Design review of the part built by this model. Coordinates are the model's own, in mm. A direction names the side the tool comes from. Round coordinates to 2 decimals unless told otherwise and drop trailing zeros. Loops run counter-clockwise (first coordinate to the right, second up) from the corner with the lowest first, then second, coordinate; pieces in that order, holes last. Notation, with made-up numbers: (-3, 21) -> (16, 21) arc R20 ccw to (16, 52) -> close; hole circle Ø4 at (-17.75, -30). An arc over 180 degrees is marked (long way). Answer as CSV lines item,"result". Start each with the question number.
(1) Draft analysis for pull direction X (two halves, no side actions). For faces 5 (the face through (-37.82, 50.91, -0.44)), 6 (the face through (-83.683, 80.085, 1.014)), 7 (the face through (-135.546, 50, -1)), state which applies: +X half, -X half, draft (parallel to the pull), parting line (faces both ways), or undercut.
(2) Take a section at A-A, the plane x = -70. Write out the cut boundary in (y, z).
(3) Take a section at B-B, the plane z = 0.95. State how many separate pieces and enclosed holes the cut face has, and give its area (3 significant figures).
(4) Take a section at C-C, the plane x = -91.5. Write out the cut boundary in (y, z), and give its area (3 significant figures).
(5) Take a section at D-D, the plane y = 74.5. Write out the cut boundary in (x, z).
(6) To check wall thickness, follow line 1 (X direction, y = 63.5, z = -1.85); line 2 (X direction, y = 53.5, z = 1.3); line 3 (X direction, y = 65, z = 0.1). State the ranges of each line that lie inside material, in increasing order. Write a range as from..to.
(7) For P1, Ø1, axis at y = 63.5, z = -2.5, coming from the +X side; P2, Ø5.5, axis at x = -103.53, y = 78.4, coming from the +Z side; P3, Ø1, axis at x = -108.5, z = 1.5, coming from the -Y side; P4, Ø1.5, axis at x = -127.5, z = -0.5, coming from the +Y side, all flat-tipped, find the tip position at first contact; note any pin that passes through.
(8) Machinability: for faces 1 (the face through (-92, 51, 0)), 2 (the face through (-117.68, 67, -1)), 3 (the face through (-84, 76, 0)), 4 (the face through (-83.486, 51, 1)), which of the approach directions +Z, -Z, +X, -X, +Y, -Y give a long, thin tool a straight path to every point of the face, cutting with its end or side? Answer none if there is none.
from build123d import *

# Parameters (mm, degrees)
ESQUISSE1_R             = 1.7
BOSS_EXTRU_1_DEPTH      = 3
ESQUISSE2_R             = 5.2
BOSS_EXTRU_2_DEPTH      = 3
BOSS_EXTRU_2_DEPTH_BACK = 3
ESQUISSE5_W             = 129.390100882
ESQUISSE5_H             = 120.053414285
ENL_V_MAT_EXTRU_2_DEPTH = 1
ESQUISSE6_R             = 1.5
ENL_V_MAT_EXTRU_3_DEPTH = 8
ESQUISSE7_W             = 14.610679854
ESQUISSE7_H             = 62.75
ENL_V_MAT_EXTRU_4_DEPTH = 8
BOSS_EXTRU_3_DEPTH      = 7
BOSS_EXTRU_4_DEPTH      = 7
ESQUISSE11_W            = 149.051338644
ESQUISSE11_H            = 13.366564364
ENL_V_MAT_EXTRU_5_DEPTH = 80
ESQUISSE13_R            = 1.7
ENL_V_MAT_EXTRU_6_DEPTH = 15


with BuildPart() as part:
    # Esquisse1 → Boss.-Extru.1 (new body)
    with BuildSketch(Plane.XY):
        with BuildLine():
            Line((-117.680084405, 66.939310237), (-117.680084405, 59.695120061))
            ThreePointArc((-117.680084405, 59.695120061), (-116.069171702, 55.806032765), (-112.180084405, 54.195120061))
            Line((-112.180084405, 54.195120061), (-105.294175096, 54.195120061))
            ThreePointArc((-105.294175096, 54.195120061), (-101.4050878, 52.584207358), (-99.794175096, 48.695120061))
            Line((-99.794175096, 48.695120061), (-99.794175096, 35.930823665))
            ThreePointArc((-99.794175096, 35.930823665), (-101.4050878, 32.041736368), (-105.294175096, 30.430823665))
            Line((-105.294175096, 30.430823665), (-112.180084405, 30.430823665))
            ThreePointArc((-112.180084405, 30.430823665), (-116.069171702, 28.819910961), (-117.680084405, 24.930823665))
            Line((-117.680084405, 24.930823665), (-117.680084405, 23.910007682))
            ThreePointArc((-117.680084405, 23.910007682), (-116.069171702, 20.020920385), (-112.180084405, 18.410007682))
            Line((-112.180084405, 18.410007682), (-105.294175096, 18.410007682))
            ThreePointArc((-105.294175096, 18.410007682), (-101.4050878, 16.799094979), (-99.794175096, 12.910007682))
            Line((-99.794175096, 12.910007682), (-99.794175096, 1.692208933))
            ThreePointArc((-99.794175096, 1.692208933), (-101.4050878, -2.196878364), (-105.294175096, -3.807791067))
            Line((-105.294175096, -3.807791067), (-113.390601299, -3.807791067))
            ThreePointArc((-113.390601299, -3.807791067), (-117.279688595, -5.418703771), (-118.890601299, -9.307791067))
            Line((-118.890601299, -9.307791067), (-118.890601299, -18.42196685))
            ThreePointArc((-118.890601299, -18.42196685), (-117.279688595, -22.311054147), (-113.390601299, -23.92196685))
            Line((-113.390601299, -23.92196685), (-52.866544484, -23.92196685))
            ThreePointArc((-52.866544484, -23.92196685), (-48.977457187, -22.311054147), (-47.366544484, -18.42196685))
            Line((-47.366544484, -18.42196685), (-47.366544484, -9.307791067))
            ThreePointArc((-47.366544484, -9.307791067), (-48.977457187, -5.418703771), (-52.866544484, -3.807791067))
            Line((-52.866544484, -3.807791067), (-77.986378892, -3.807791067))
            ThreePointArc((-77.986378892, -3.807791067), (-81.875466189, -2.196878364), (-83.486378892, 1.692208933))
            Line((-83.486378892, 1.692208933), (-83.486378892, 12.910007682))
            ThreePointArc((-83.486378892, 12.910007682), (-81.875466189, 16.799094979), (-77.986378892, 18.410007682))
            Line((-77.986378892, 18.410007682), (-69.856378892, 18.410007682))
            ThreePointArc((-69.856378892, 18.410007682), (-65.967291596, 20.020920385), (-64.356378892, 23.910007682))
            Line((-64.356378892, 23.910007682), (-64.356378892, 24.930823665))
            ThreePointArc((-64.356378892, 24.930823665), (-65.967291596, 28.819910961), (-69.856378892, 30.430823665))
            Line((-69.856378892, 30.430823665), (-77.986378892, 30.430823665))
            ThreePointArc((-77.986378892, 30.430823665), (-81.875466189, 32.041736368), (-83.486378892, 35.930823665))
            Line((-83.486378892, 35.930823665), (-83.486378892, 55.219310237))
            ThreePointArc((-83.486378892, 55.219310237), (-81.875466189, 59.108397534), (-77.986378892, 60.719310237))
            Line((-77.986378892, 60.719310237), (-54.190366806, 60.719310237))
            ThreePointArc((-54.190366806, 60.719310237), (-50.30127951, 62.330222941), (-48.690366806, 66.219310237))
            Line((-48.690366806, 66.219310237), (-48.690366806, 67.219310237))
            Line((-48.690366806, 67.219310237), (-48.690366806, 77.901748252))
            ThreePointArc((-48.690366806, 77.901748252), (-50.30127951, 81.790835548), (-54.190366806, 83.401748252))
            Line((-54.190366806, 83.401748252), (-112.180084405, 83.401748252))
            ThreePointArc((-112.180084405, 83.401748252), (-116.069171702, 81.790835548), (-117.680084405, 77.901748252))
            Line((-117.680084405, 77.901748252), (-117.680084405, 67.219310237))
            Line((-117.680084405, 67.219310237), (-117.680084405, 66.939310237))
        make_face()
        with Locations((-59.266378892, -15.663707737)):
            Circle(ESQUISSE1_R, mode=Mode.SUBTRACT)
        with Locations((-59.266378892, 66.939310237)):
            Circle(ESQUISSE1_R, mode=Mode.SUBTRACT)
        with Locations((-91.856378892, 36.719310237)):
            Circle(ESQUISSE1_R, mode=Mode.SUBTRACT)
        with Locations((-107.466378892, -14.520689763)):
            Circle(ESQUISSE1_R, mode=Mode.SUBTRACT)
        with Locations((-107.466378892, 60.719310237)):
            Circle(ESQUISSE1_R, mode=Mode.SUBTRACT)
        with Locations((-58.306378892, 78.399310237)):
            Circle(ESQUISSE1_R, mode=Mode.SUBTRACT)
        with Locations((-108.486378892, 78.399310237)):
            Circle(ESQUISSE1_R, mode=Mode.SUBTRACT)
        with BuildLine():
            Line((-111.390601299, 21.460065469), (-70.086378892, 21.460065469))
            ThreePointArc((-70.086378892, 21.460065469), (-68.67216533, 22.045851906), (-68.086378892, 23.460065469))
            Line((-68.086378892, 23.460065469), (-68.086378892, 24.842520386))
            ThreePointArc((-68.086378892, 24.842520386), (-68.67216533, 26.256733949), (-70.086378892, 26.842520386))
            Line((-70.086378892, 26.842520386), (-111.390601299, 26.842520386))
            ThreePointArc((-111.390601299, 26.842520386), (-112.804814861, 26.256733949), (-113.390601299, 24.842520386))
            Line((-113.390601299, 24.842520386), (-113.390601299, 23.460065469))
            ThreePointArc((-113.390601299, 23.460065469), (-112.804814861, 22.045851906), (-111.390601299, 21.460065469))
        make_face(mode=Mode.SUBTRACT)
    extrude(amount=BOSS_EXTRU_1_DEPTH)

    # Esquisse2 → Boss.-Extru.2 (add, two sides)
    with BuildSketch(Plane(origin=(0, 0, 0), x_dir=(-1, 0, 0), z_dir=(0, 0, -1))) as boss_extru_2_sk:
        with BuildLine():
            Line((118.890601299, -9.969506719), (130.584615963, -9.880075131))
            ThreePointArc((130.584615963, -9.880075131), (134.095405897, -8.402210456), (135.546378892, -4.880221341))
            Line((135.546378892, -4.880221341), (135.546378892, 5.415623015))
            ThreePointArc((135.546378892, 5.415623015), (136.425058549, 7.536943358), (138.546378892, 8.415623015))
            Line((138.546378892, 8.415623015), (145.752654566, 8.415623015))
            ThreePointArc((145.752654566, 8.415623015), (147.87397491, 9.294302671), (148.752654566, 11.415623015))
            Line((148.752654566, 11.415623015), (148.752654566, 38.179170847))
            ThreePointArc((148.752654566, 38.179170847), (147.87397491, 40.300491191), (145.752654566, 41.179170847))
            Line((145.752654566, 41.179170847), (138.546378892, 41.179170847))
            ThreePointArc((138.546378892, 41.179170847), (136.425058549, 42.057850504), (135.546378892, 44.179170847))
            Line((135.546378892, 44.179170847), (135.546378892, 52.099902349))
            ThreePointArc((135.546378892, 52.099902349), (134.081912798, 55.635436255), (130.546378892, 57.099902349))
            Line((130.546378892, 57.099902349), (117.680084405, 57.099902349))
            Line((117.680084405, 57.099902349), (117.680084405, 72.719310237))
            Line((117.680084405, 72.719310237), (48.690366806, 72.719310237))
            Line((48.690366806, 72.719310237), (48.690366806, 60.719310237))
            Line((48.690366806, 60.719310237), (48.690366806, 57.099902349))
            Line((48.690366806, 57.099902349), (40.256901013, 57.099902349))
            ThreePointArc((40.256901013, 57.099902349), (37.428473888, 55.928329474), (36.256901013, 53.099902349))
            Line((36.256901013, 53.099902349), (36.256901013, 47.456292263))
            Line((36.256901013, 47.456292263), (39.346378892, 47.456292263))
            ThreePointArc((39.346378892, 47.456292263), (41.396631424, 52.406039732), (46.346378892, 54.456292263))
            Line((46.346378892, 54.456292263), (126.246378892, 54.456292263))
            ThreePointArc((126.246378892, 54.456292263), (131.196126361, 52.406039732), (133.246378892, 47.456292263))
            Line((133.246378892, 47.456292263), (133.246378892, 40.977229779))
            ThreePointArc((133.246378892, 40.977229779), (134.125058549, 38.855909436), (136.246378892, 37.977229779))
            Line((136.246378892, 37.977229779), (142.162261637, 37.977229779))
            ThreePointArc((142.162261637, 37.977229779), (144.28358198, 37.098550123), (145.162261637, 34.977229779))
            Line((145.162261637, 34.977229779), (145.162261637, 14.363062522))
            ThreePointArc((145.162261637, 14.363062522), (144.28358198, 12.241742179), (142.162261637, 11.363062522))
            Line((142.162261637, 11.363062522), (136.246378892, 11.363062522))
            ThreePointArc((136.246378892, 11.363062522), (134.125058549, 10.484382866), (133.246378892, 8.363062522))
            Line((133.246378892, 8.363062522), (133.246378892, -1.293707737))
            ThreePointArc((133.246378892, -1.293707737), (131.196126361, -6.243455205), (126.246378892, -8.293707737))
            Line((126.246378892, -8.293707737), (46.346378892, -8.293707737))
            ThreePointArc((46.346378892, -8.293707737), (41.396631424, -6.243455205), (39.346378892, -1.293707737))
            Line((39.346378892, -1.293707737), (36.248203357, -1.293707737))
            Line((36.248203357, -1.293707737), (36.248203357, -6.64542392))
            ThreePointArc((36.248203357, -6.64542392), (37.432020164, -9.486042202), (40.282759469, -10.645274652))
            Line((40.282759469, -10.645274652), (47.366544484, -10.58407535))
            Line((47.366544484, -10.58407535), (47.366544484, -23.92196685))
            Line((47.366544484, -23.92196685), (118.890601299, -23.92196685))
            Line((118.890601299, -23.92196685), (118.890601299, -9.969506719))
        make_face()
        with Locations((59.266378892, -15.663707737)):
            Circle(ESQUISSE2_R, mode=Mode.SUBTRACT)
        with Locations((107.466378892, -14.520689763)):
            Circle(ESQUISSE2_R, mode=Mode.SUBTRACT)
        with Locations((107.466378892, 60.719310237)):
            Circle(ESQUISSE2_R, mode=Mode.SUBTRACT)
        with Locations((59.266378892, 66.939310237)):
            Circle(ESQUISSE2_R, mode=Mode.SUBTRACT)
    extrude(amount=BOSS_EXTRU_2_DEPTH)
    extrude(boss_extru_2_sk.sketch, amount=-BOSS_EXTRU_2_DEPTH_BACK)

    # Esquisse5 → Enl_v. mat.-Extru.2 (cut)
    with BuildSketch(Plane.XY.offset(3)):
        with Locations((-91.695706627, 29.828971757)):
            Rectangle(ESQUISSE5_W, ESQUISSE5_H)
    extrude(amount=-ENL_V_MAT_EXTRU_2_DEPTH, mode=Mode.SUBTRACT)

    # Esquisse6 → Enl_v. mat.-Extru.3 (cut)
    with BuildSketch(Plane.XY.offset(2)):
        with Locations((-69.623492164, 64.727424081)):
            Circle(ESQUISSE6_R)
        with Locations((-83.623492164, 64.727424081)):
            Circle(ESQUISSE6_R)
    extrude(amount=-ENL_V_MAT_EXTRU_3_DEPTH, mode=Mode.SUBTRACT)

    # Esquisse7 → Enl_v. mat.-Extru.4 (cut)
    with BuildSketch(Plane(origin=(0, 0, 0), x_dir=(-1, 0, 0), z_dir=(0, 0, -1))):
        with Locations((42.567758063, 23.081292263)):
            Rectangle(ESQUISSE7_W, ESQUISSE7_H)
    extrude(amount=ENL_V_MAT_EXTRU_4_DEPTH, mode=Mode.SUBTRACT)

    # Esquisse9 → Boss.-Extru.3 (add)
    with BuildSketch(Plane(origin=(0, -1.293707737, 0), x_dir=(1, 0, 0), z_dir=(0, 1, 0))):
        Polygon((-39.346378892, -2), (-39.346378892, 0.886005049), (-36.248203357, 0), (-36.248203357, -2), align=None)
    extrude(amount=-BOSS_EXTRU_3_DEPTH)

    # Esquisse10 → Boss.-Extru.4 (add)
    with BuildSketch(Plane.XZ.offset(-47.456292263)):
        Polygon((-39.346378892, 2), (-39.346378892, -0.873043126), (-36.256901013, 0), (-36.256901013, 2), align=None)
    extrude(amount=-BOSS_EXTRU_4_DEPTH)

    # Esquisse11 → Enl_v. mat.-Extru.5 (cut)
    with BuildSketch(Plane.XZ.offset(-47.456292263)):
        with Locations((-92.889015797, -0.494206667)):
            Rectangle(ESQUISSE11_W, ESQUISSE11_H)
    extrude(amount=ENL_V_MAT_EXTRU_5_DEPTH, mode=Mode.SUBTRACT)

    # Esquisse13 → Enl_v. mat.-Extru.6 (cut)
    with BuildSketch(Plane.XY.offset(2)):
        with Locations((-103.52911982, 78.399310237)):
            Circle(ESQUISSE13_R)
        with Locations((-88.23911982, 78.399310237)):
            Circle(ESQUISSE13_R)
        with Locations((-83.462080633, 78.399310237)):
            Circle(ESQUISSE13_R)
        with Locations((-64.462080633, 78.399310237)):
            Circle(ESQUISSE13_R)
    extrude(amount=-ENL_V_MAT_EXTRU_6_DEPTH, mode=Mode.SUBTRACT)


solid = part.part
The answers:
1,face 5,"+X half"
1,face 6,"undercut"
1,face 7,"-X half"
2,outline,"(54.46, -3) -> (63.28, -3) -> (63.28, 2) -> (54.46, 2) -> close; (66.18, -3) -> (72.72, -3) -> (72.72, 0) -> (83.4, 0) -> (83.4, 2) -> (66.18, 2) -> close"
3,separate pieces,"1"
3,enclosed holes,"10"
3,area,"2,150 mm²"
4,outline,"(47.46, 0) -> (54.46, 0) -> (54.46, -3) -> (72.72, -3) -> (72.72, 0) -> (83.4, 0) -> (83.4, 2) -> (47.46, 2) -> close"
4,area,"127 mm²"
5,outline,"(-117.68, 0) -> (-48.69, 0) -> (-48.69, 2) -> (-117.68, 2) -> close"
6,line 1,"-117.68..-111.86, -103.07..-84.49, -82.76..-70.49, -68.76..-63.17, -55.37..-48.69"
6,line 2,"-135.35..-129.78, -102.62..-83.49, -42.81..-36.26"
6,line 3,"-117.68..-85.1, -82.15..-71.1, -68.15..-48.69"
7,P1,"x = -48.69"
7,P2,"z = 2"
7,P3,"y = 54.2"
7,P4,"y = 57.1"
8,face 1,"-Z, -Y"
8,face 2,"+Z, -Z, -X, +Y"
8,face 3,"-Z, +X, -X, +Y"
8,face 4,"+Z, -Z, -Y"
